from build123d import *

# Parameters (mm, degrees)
CHAMFER1_SIZE      = 0.8
CUT_EXTRUDE1_DEPTH = 6


with BuildPart() as part:
    # Sketch1 → Revolve1 (revolve)
    with BuildSketch(Plane.XY):
        Polygon((0, 0), (0, 5.582013072), (0.53, 6.5), (7.47, 6.5), (8, 5.582013072), (8, 4), (38, 4), (38, 0), align=None)
    revolve(axis=Axis((38, 0, 0), (-1, 0, 0)))

    # Chamfer1
    chamfer1_edges = [part.edges().sort_by_distance(p)[0] for p in [
        (38, -4, 0),
    ]]
    chamfer(chamfer1_edges, length=CHAMFER1_SIZE)

    # Sketch2 → Cut-Extrude1 (cut)
    with BuildSketch(Plane.ZY):
        Polygon((3.75277675, 0), (1.876388375, 3.25), (-1.876388375, 3.25), (-3.75277675, 0), (-1.876388375, -3.25), (1.876388375, -3.25), align=None)
    extrude(amount=-CUT_EXTRUDE1_DEPTH, mode=Mode.SUBTRACT)

    # Sketch4 → Cut-Revolve1 (revolve, cut)
    with BuildSketch(Plane.XY, mode=Mode.PRIVATE) as cut_revolve1_sk:
        Polygon((0, 0), (0, 4), (2.309401077, 0), align=None)
        Polygon((6, 0), (6, 4), (8.309401077, 0), align=None)
    revolve(cut_revolve1_sk.sketch.rotate(Axis((0, 0, 0), (1, 0, 0)), 90), axis=Axis((0, 0, 0), (1, 0, 0)), mode=Mode.SUBTRACT)


solid = part.part
For this review, take the finished solid that the model builds, in its own axes (mm). A direction names the side the tool comes from. Round coordinates to 2 decimals unless told otherwise and drop trailing zeros. Order: outer loops, then holes, each group sorted by start corner. A loop starts at its lowest first (then second) coordinate and runs counter-clockwise, first axis right, second up. Notation, with made-up numbers: (81, -6) -> (113, -6) arc R32 ccw to (113, 24) -> close; hole circle Ø3 at (38, 24). An arc over 180 degrees is marked (long way). Write item = value, one per line. Start each with the question number.
1) Take a section at A-A on x = 3.5. State the section outline as (y, z) points.
2) Tool access review of faces 1 (the face through (38, 0, 0)), 2 (the face through (6, -2, -3)), 3 (the face through (3, -3.25, 0)), 4 (the face through (22.804, -0.867, 3.905)): name each direction out of +Z, -Z, +X, -X, +Y, -Y from which nothing blocks a thin tool from reaching the whole face with its end or side.
3) Insertion check: pin 1 (6 mm diameter, centred on x = 16.5, y = -3.5, fed in from -Z); pin 2 (1.5 mm diameter, centred on x = 24.5, z = 1.5, fed in from -Y); pin 3 (3 mm diameter, centred on y = -3, z = -4.5, fed in from +X). Each pin has a flat end and moves straight along its axis. Give the tip position at first contact, or say it passes through.
4) The part is to be moulded in two halves that separate along Y. For faces 5 (the face through (3.03, -1.65, 2.8)), 6 (the face through (4.049, -5.158, 3.955)), 7 (the face through (0, -2, 4)), say which applies: +Y half, -Y half, draft (parallel to the pull), parting line (faces both ways), or undercut.
5) To check wall thickness, follow line 1 (X direction, y = 4.5, z = 1.25); line 2 (Z direction, x = 26.5, y = 0); line 3 (Y direction, x = 32, z = 0.25). State the ranges of each line that lie inside material, in increasing order. Write a range as from..to.
6) Take a section at B-B on x = 34.5. State the section outline as (y, z) points.
Verdict:
q1.outline = circle Ø13 at (0, 0); hole (-3.25, -1.88) -> (0, -3.75) -> (3.25, -1.88) -> (3.25, 1.88) -> (0, 3.75) -> (-3.25, 1.88) -> close
q2.face_1 = +Z, -Z, +X, +Y, -Y
q2.face_2 = none
q2.face_3 = -X
q2.face_4 = +X
q3.pin_1 = -3.97
q3.pin_2 = -3.93
q3.pin_3 = 37.29
q4.face_5 = undercut
q4.face_6 = parting line
q4.face_7 = draft
q5.line_1 = 0..8
q5.line_2 = -4..4
q5.line_3 = -3.99..3.99
q6.outline = circle Ø8 at (0, 0)
